Here's how the part is built. I have some questions about the finished solid (model axes, mm). A direction names the side the tool comes from. Coordinates: 2 decimals unless noted, no trailing zeros. Loops run counter-clockwise (first coordinate to the right, second up) from the corner with the lowest first, then second, coordinate; pieces in that order, holes last. Notation, with made-up numbers: (31.5, 36) - (54.5, 36) arc R16 cw to (54.5, 54) - close; hole circle Ø7 at (9, 25). An arc over 180 degrees is marked (long way). Use a Markdown table: item, result.
```python
from build123d import *

# Parameters (mm, degrees)
F0_W       = 38.1
F0_H       = 152.4
F1_DEPTH   = 6.35
F2_SIZE2   = 2.53999
F2_SIZE    = 6.34999
F2_2_SIZE2 = 2.53999
F2_2_SIZE  = 6.34999
F3_W       = 152.4
F3_H       = 6.8391593051
F4_DEPTH   = 10.16
F5_W       = 152.4
F5_H       = 6.8391593051
F6_DEPTH   = 10.16
F7_R       = 3.81
F8_W       = 31.75
F8_H       = 5.08
F9_DEPTH   = 6.35
F10_W      = 4.318
F10_H      = 26.67
F11_DEPTH  = 25.4
F12_R      = 1.016
F13_R      = 14.3701538506
F14_DEPTH  = 2.54


# Not quite as in the source:
# - a fillet or chamfer is up to 0.001 mm smaller than in the source, because OpenCascade refuses the exact size


with BuildPart() as f1:
    # F0 (on Top) → F1 (new body)
    with BuildSketch(Plane.XY):
        with Locations((0.2864310518, 39.6771576124)):
            Rectangle(F0_W, F0_H)
    extrude(amount=F1_DEPTH)

    # F2 (size 6.35 and 2.54 in the source; OpenCascade refuses exactly that, so slightly less here)
    f2_edges = [f1.edges().sort_by_distance(p)[0] for p in [
        (-18.763569, 39.677158, 0),
    ]]
    f2_side = f1.faces().sort_by_distance((-18.763569, 39.677158, 3.175))[0]
    chamfer(f2_edges, length=F2_SIZE, length2=F2_SIZE2, reference=f2_side)

    # F2#2 (size 6.35 and 2.54 in the source; OpenCascade refuses exactly that, so slightly less here)
    f2_2_edges = [f1.edges().sort_by_distance(p)[0] for p in [
        (19.336431, 39.677158, 0),
    ]]
    f2_2_side = f1.faces().sort_by_distance((19.336431, 39.677158, 3.175))[0]
    chamfer(f2_2_edges, length=F2_2_SIZE, length2=F2_2_SIZE2, reference=f2_2_side)

    # F3 (on face) → F4 (join)
    with BuildSketch(Plane(origin=(-13.9858353002, 0, -5.5943341201), x_dir=(0, -1, 0), z_dir=(-0.9284766909, 0, -0.3713906764))):
        with Locations((-39.6771576124, 9.4448618971)):
            Rectangle(F3_W, F3_H)
    extrude(amount=F4_DEPTH)

    # F5 (on face) → F6 (join)
    with BuildSketch(Plane(origin=(14.4796819412, 0, -5.7918727765), x_dir=(0, 1, 0), z_dir=(0.9284766909, 0, -0.3713906764))):
        with Locations((39.6771576124, 9.6576175412)):
            Rectangle(F5_W, F5_H)
    extrude(amount=F6_DEPTH)

    # F7
    f7_edges = [f1.edges().sort_by_distance(p)[0] for p in [
        (0.286431, -36.522842, 0),
        (-20.940231, -36.522842, -1.886665),
        (21.513093, -36.522842, -1.886665),
        (21.513093, 115.877158, -1.886665),
        (0.286431, 115.877158, 0),
        (-20.940231, 115.877158, -1.886665),
    ]]
    fillet(f7_edges, radius=F7_R)

    # F8 (on face) → F9 (join)
    with BuildSketch(Plane(origin=(-23.4191584796, 0, -9.3676633918), x_dir=(0, -1, 0), z_dir=(-0.9284766909, 0, -0.3713906764))):
        with Locations((-87.9551129937, 8.5652822446)):
            Rectangle(F8_W, F8_H)
    extrude(amount=F9_DEPTH)

    # F10 (on face) → F11 (cut)
    with BuildSketch(Plane(origin=(-4.1243982839, 0, 10.3109957098), x_dir=(0.9284766909, 0, 0.3713906764), z_dir=(-0.3713906764, 0, 0.9284766909))):
        with Locations((-27.3822056114, 87.9551129937)):
            Rectangle(F10_W, F10_H)
    extrude(amount=-F11_DEPTH, mode=Mode.SUBTRACT)

    # F12
    f12_edges = [f1.edges().sort_by_distance(p)[0] for p in [
        (-31.552719, 87.955113, -0.660333),
        (-29.666054, 87.955113, -5.376994),
    ]]
    fillet(f12_edges, radius=F12_R)

    # F13 (on face) → F14 (join)
    with BuildSketch(Plane.XY.offset(6.35)):
        with Locations((0, 87.3177349567)):
            Circle(F13_R)
    extrude(amount=F14_DEPTH)


solid = f1.part
```
Q1. I want a section at C-C, the plane y = -24.5. Write out the boundary of the cut face in (x, z), then the cut area to 3 significant figures.
Check values:
| item | result |
|---|---|
| outline | (-28.2, 2.58) - (-25.66, -3.77) - (-16.22, 0) - (16.8, 0) - (26.23, -3.77) - (28.77, 2.58) - (19.34, 6.35) - (-18.76, 6.35) - close |
| area | 365 mm^2 |
Q2. I want a section at A-A, the plane y = 80. Write out the boundary of the cut face in (x, z) (3 decimals).
Check values:
| item | result |
|---|---|
| outline | (-33.439, -1.415) - (-31.553, -6.132) - (-30.609, -5.754) arc R1.016 ccw to (-30.043, -4.434) - (-31.175, -1.604) arc R1.016 ccw to (-32.496, -1.038) - close; (-28.197, 2.577) - (-25.657, -3.773) - (-16.224, 0) - (16.796, 0) - (26.23, -3.773) - (28.77, 2.577) - (19.336, 6.35) - (12.367, 6.35) - (12.367, 8.89) - (-12.367, 8.89) - (-12.367, 6.35) - (-18.764, 6.35) - close |
Q3. I want a section at B-B, the plane x = 0. Write out the boundary of the cut face in (y, z).
Check values:
| item | result |
|---|---|
| outline | (-36.52, 3.81) arc R3.81 ccw to (-32.71, 0) - (112.07, 0) arc R3.81 ccw to (115.88, 3.81) - (115.88, 6.35) - (101.69, 6.35) - (101.69, 8.89) - (72.95, 8.89) - (72.95, 6.35) - (-36.52, 6.35) - close |
Q4. Please list where these lines run through material, in increasing order: L1, parallel to X at y = 91.5, z = -1.5; L2, parallel to Z at x = 9, y = -2; L3, parallel to X at y = 4.5, z = 2.5. Write a range as from..to.
Check values:
| item | result |
|---|---|
| L1 | -33.41..-31.22, -26.57..-19.97, 20.55..27.14 |
| L2 | 0..6.35 |
| L3 | -28.17..28.74 |
Q5. Which directions (+Z, -Z, +X, -X, +Y, -Y) give clear straight access to the entire face, cutting with the end or side of a thin tool? Please do faces 1 (the face through (0.53, -35.44, 1.15)), 2 (the face through (-21.096, 114.791, -0.715)), 3 (the face through (0, 41, 0)), 4 (the face through (-29, 72.08, -3)).
Check values:
| item | result |
|---|---|
| face 1 | -Z, -Y |
| face 2 | -Z, +Y |
| face 3 | -Z, +Y, -Y |
| face 4 | -Z, -X, -Y |
Q6. Will these pins go through, and if not, where does the flat tip stop? P1, Ø1, axis at x = 3, y = -5, coming from the +Z side; P2, Ø10, axis at x = -4.5, y = 53.5, coming from the -Z side; P3, Ø4, axis at y = 69.5, z = -3.5, coming from the +X side.
Check values:
| item | result |
|---|---|
| P1 | z = 6.35 |
| P2 | z = 0 |
| P3 | x = 27.14 |
Q7. If we mould it in two halves opening along X, with no side actions, what happens to faces 5 (the face through (-1, -36.523, 5)), 6 (the face through (23.99, 38.61, 4.49)), 7 (the face through (-29, 74.62, -2)), 8 (the face through (21.67, -35.44, -0.71))? For each: pulls with the +X half, pulls with the -X half, needs draft (parallel to the pull), parting line crosses it, or undercut.
Check values:
| item | result |
|---|---|
| face 5 | needs draft |
| face 6 | pulls with the +X half |
| face 7 | undercut |
| face 8 | undercut |
